Design review of the part shown in the three views and the two pictorial views. Dimensions are in mm from the part's minimum x, y and z. A direction names the side the tool comes from. Give positions to 0.01 mm unless a question says otherwise; leave off trailing zeros. Order: outer loops, then holes, each group sorted by start corner. A loop starts at its lowest first (then second) coordinate and runs counter-clockwise, first axis right, second up. Notation, with made-up numbers: (52, 36) -> (82, 36) arc R23 ccw to (82, 54) -> close; hole circle Ø5 at (-10.75, 66). An arc over 180 degrees is marked (long way). Use one line per item in the form item = value.
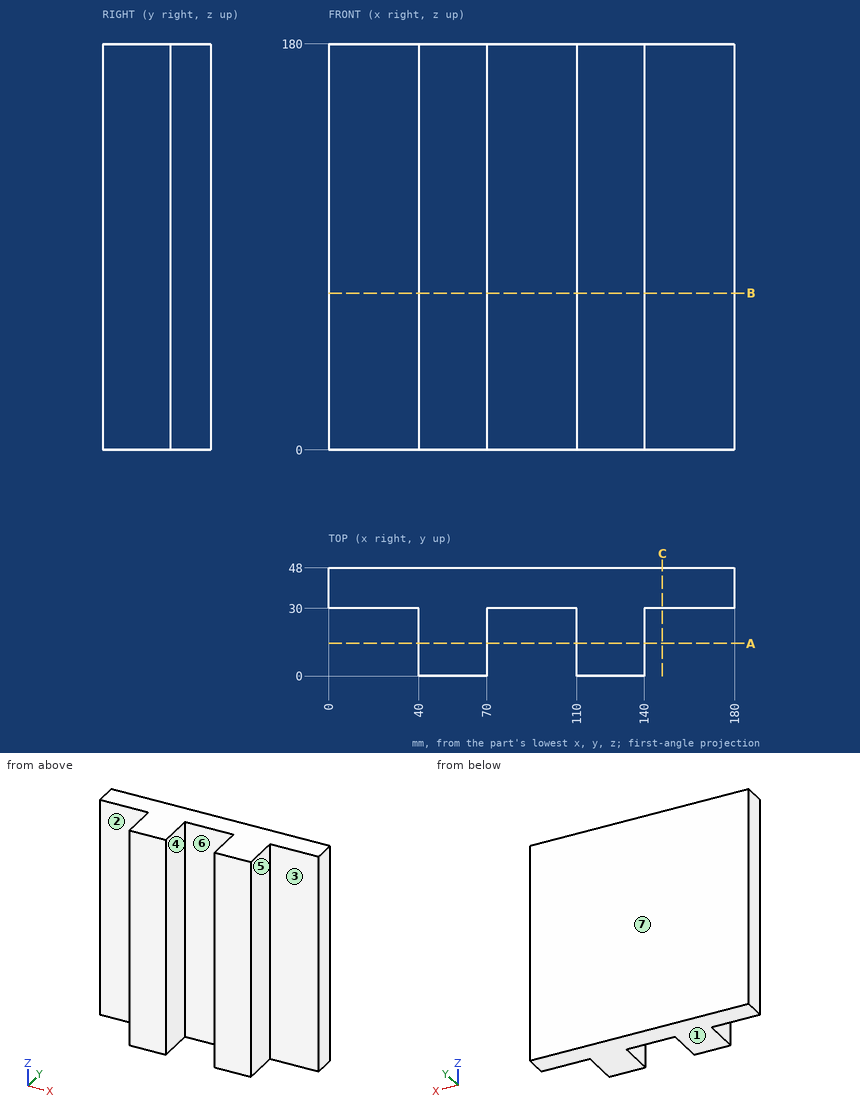
1. Add section A-A on y = 14.5. Give the boundary of the cut face in (x, z).
Values:
outline = (40, 0) -> (70, 0) -> (70, 180) -> (40, 180) -> close; (110, 0) -> (140, 0) -> (140, 180) -> (110, 180) -> close
2. For L1, parallel to X at y = 6.5, z = 96; L2, parallel to Y at x = 83, z = 108.5, list the stretches that pass through material, from the lowest coordinate up.
Values:
L1 = 40 to 70, 110 to 140
L2 = 30 to 48
3. The part is to be moulded in two halves that separate along X. For the marked faces 5, 6 and 7, say which applies: +X half, -X half, draft (parallel to the pull), parting line (faces both ways), or undercut.
Values:
face_5 = +X half
face_6 = undercut
face_7 = draft
4. Add section B-B on z = 69.5. Give the boundary of the cut face in (x, y).
Values:
outline = (0, 30) -> (40, 30) -> (40, 0) -> (70, 0) -> (70, 30) -> (110, 30) -> (110, 0) -> (140, 0) -> (140, 30) -> (180, 30) -> (180, 48) -> (0, 48) -> close
5. Add section C-C on x = 148. Give the boundary of the cut face in (y, z), then the cut area to 3 significant figures.
Values:
outline = (30, 0) -> (48, 0) -> (48, 180) -> (30, 180) -> close
area = 3,240 mm^2
6. For pin 1 Ø9 at (y, z) = (14, 94.5) entering from -X; pin 2 Ø12 at (x, z) = (88.5, 120) entering from -Y; pin 3 Ø6 at (x, y) = (41, 27) entering from -Z; pin 4 Ø9 at (y, z) = (10, 71) entering from +X, all flat-tipped, find the tip position at first contact; note any pin that passes through.
Values:
pin_1 = 40
pin_2 = 30
pin_3 = 0
pin_4 = 140
7. Tool access review of the marked faces 1, 2, 3 and 4: name each direction out of +Z, -Z, +X, -X, +Y, -Y from which nothing blocks a thin tool from reaching the whole face with its end or side.
Values:
face_1 = -Z, +X, -X, +Y, -Y
face_2 = +Z, -Z, -X, -Y
face_3 = +Z, -Z, +X, -Y
face_4 = +Z, -Z, -Y
